The listing builds one solid part. Answer for the finished solid, in the listing's coordinates (mm). A direction names the side the tool comes from. Coordinates: 2 decimals unless noted, no trailing zeros. Write each loop counter-clockwise with the first axis right and the second up, starting at its lowest first coordinate (ties: lowest second). Pieces come first, ordered by that corner, then holes.
(1) Given P1, Ø0.9, axis at y = -12, z = 5, coming from the -X side; P2, Ø2, axis at y = -8.5, z = 1.5, coming from the +X side; P3, Ø1.5, axis at x = 30, z = 4, coming from the -Y side, each flat-ended and moving along its own axis, determine where each tip first touches the part or whether it passes through.
(2) The part is cut by section C-C on y = -26. Determine the outline of the cut face in (x, z), plus the area to 3 significant figures.
(3) Straight lines are drawn through the part: line 1 (Y direction, x = 7.5, z = 1.8); line 2 (Z direction, x = 4, y = -27); line 3 (Y direction, x = 27, z = 4.3). For each, find the intervals that lie inside material, in ascending order.
(4) The part is cut by section B-B on x = 7.5. Determine the outline of the cut face in (y, z), plus the area to 3 significant figures.
(5) Which of the six approach directions +Z, -Z, +X, -X, +Y, -Y give full straight-line access (tool end or side, diameter ignored) to faces 1 (the flat face through (12, -15, 4)), 2 (the cylindrical face through (14.699, -4.451, 2.715)), 3 (the cylindrical face through (14.699, -25.451, 2.715))?
(6) The part is cut by section D-D on z = 2.55. Determine the outline of the cut face in (x, y), plus the area to 3 significant figures.
(7) The part is cut by section A-A on y = -22.5. Determine the outline of the cut face in (x, z), plus the area to 3 significant figures.
from build123d import *

# Parameters (mm, degrees)
SKETCH1_W           = 15
SKETCH1_H           = 30
SKETCH1_R           = 2.25
BOSS_EXTRUDE1_DEPTH = 3
SKETCH3_W           = 3
SKETCH3_H           = 14
BOSS_EXTRUDE2_DEPTH = 3
SKETCH4_W           = 3
SKETCH4_H           = 14
BOSS_EXTRUDE3_DEPTH = 26
FILLET2_R           = 1


with BuildPart() as part:
    # Sketch1 → Boss-Extrude1 (new body)
    with BuildSketch(Plane.XY):
        with Locations((7.5, -15)):
            Rectangle(SKETCH1_W, SKETCH1_H)
        with Locations((7.5, -7.5)):
            Circle(SKETCH1_R, mode=Mode.SUBTRACT)
        with Locations((7.5, -22.5)):
            Circle(SKETCH1_R, mode=Mode.SUBTRACT)
    extrude(amount=BOSS_EXTRUDE1_DEPTH)

    # Sketch3 → Boss-Extrude2 (add)
    with BuildSketch(Plane.ZY.offset(-15)):
        with Locations((4.5, -15)):
            Rectangle(SKETCH3_W, SKETCH3_H)
    extrude(amount=BOSS_EXTRUDE2_DEPTH)

    # Sketch4 → Boss-Extrude3 (add)
    with BuildSketch(Plane.ZY.offset(-12)):
        with Locations((4.5, -15)):
            Rectangle(SKETCH4_W, SKETCH4_H)
    extrude(amount=-BOSS_EXTRUDE3_DEPTH)

    # Fillet2
    fillet2_edges = [part.edges().sort_by_distance(p)[0] for p in [
        (7.5, -30, 3),
        (7.5, -30, 0),
        (7.5, 0, 0),
        (7.5, 0, 3),
        (0, 0, 1.5),
        (0, -15, 3),
        (0, -30, 1.5),
        (0, -15, 0),
        (15, -30, 1.5),
        (15, 0, 1.5),
        (15, -4, 3),
        (15, -26, 3),
        (15, -15, 0),
    ]]
    fillet(fillet2_edges, radius=FILLET2_R)


solid = part.part
Model answer:
1. P1: stops at x = 12
1. P2: stops at x = 15
1. P3: stops at y = -22
2. outline: (0, 1) arc R1 ccw to (1, 0) - (14, 0) arc R1 ccw to (15, 1) - (15, 2) arc R1 ccw to (14, 3) - (1, 3) arc R1 ccw to (0, 2) - close
2. area: 44.1 mm2
3. line 1: y = -30 to -24.75, -20.25 to -9.75, -5.25 to 0
3. line 2: z = 0 to 3
3. line 3: y = -22 to -8
4. outline: (-30, 1) arc R1 ccw to (-29, 0) - (-24.75, 0) - (-24.75, 3) - (-29, 3) arc R1 ccw to (-30, 2) - close; (-20.25, 0) - (-9.75, 0) - (-9.75, 3) - (-20.25, 3) - close; (-5.25, 0) - (-1, 0) arc R1 ccw to (0, 1) - (0, 2) arc R1 ccw to (-1, 3) - (-5.25, 3) - close
4. area: 62.1 mm2
5. face 1: +Z, -X, +Y, -Y
5. face 2: +Z, +X, +Y
5. face 3: +Z, +X, -Y
6. outline: (0.16, -29) arc R0.84 ccw to (1, -29.84) - (14, -29.84) arc R0.84 ccw to (14.84, -29) - (14.84, -22) - (15, -22) - (15, -8) - (14.84, -8) - (14.84, -1) arc R0.84 ccw to (14, -0.16) - (1, -0.16) arc R0.84 ccw to (0.16, -1) - close; hole circle Ø4.5 at (7.5, -22.5); hole circle Ø4.5 at (7.5, -7.5)
6. area: 405 mm2
7. outline: (0, 1) arc R1 ccw to (1, 0) - (5.25, 0) - (5.25, 3) - (1, 3) arc R1 ccw to (0, 2) - close; (9.75, 0) - (14, 0) arc R1 ccw to (15, 1) - (15, 2) arc R1 ccw to (14, 3) - (9.75, 3) - close
7. area: 30.6 mm2
